Design review of the part built by this model. Coordinates are the model's own, in mm. A direction names the side the tool comes from. Give positions to 0.01 mm unless a question says otherwise; leave off trailing zeros. Loops run counter-clockwise (first coordinate to the right, second up) from the corner with the lowest first, then second, coordinate; pieces in that order, holes last. Notation, with made-up numbers: (35, -3.75) - (84, -3.75) arc R21 cw to (84, 0.25) - close; hole circle Ø2 at (30.5, 66). An arc over 180 degrees is marked (long way). Write each question's results on one line, items separated by ' | '.
from build123d import *

# Parameters (mm, degrees)
CROQUIS1_R                   = 15
SALIENTE_EXTRUIR1_DEPTH      = 3
CROQUIS2_R                   = 8.5
SALIENTE_EXTRUIR2_DEPTH      = 65
CORTAR_EXTRUIR1_DEPTH        = 4
CORTAR_EXTRUIR1_DEPTH_BACK   = 4
CROQUIS3_W                   = 17
CROQUIS3_H                   = 53
CORTAR_EXTRUIR2_DEPTH        = 8
CORTAR_EXTRUIR2_DEPTH_BACK   = 8
CROQUIS4_R                   = 1
CUT_EXTRUDE9_DEPTH           = 2.5
CROQUIS5_W                   = 2
CROQUIS5_H                   = 15
SALIENTE_EXTRUIR3_DEPTH      = 15
CROQUIS6_R                   = 1.5
SALIENTE_EXTRUIR4_DEPTH      = 3
SALIENTE_EXTRUIR5_DEPTH      = 1.5
SALIENTE_EXTRUIR5_DEPTH_BACK = 1.5
REDONDEO2_R                  = 6
CROQUIS8_R                   = 3
CORTAR_EXTRUIR3_DEPTH        = 10
SKETCH1_W                    = 5
SKETCH1_H                    = 5
CUT_EXTRUDE1_DEPTH           = 1
SKETCH2_R                    = 1.25
CUT_EXTRUDE2_DEPTH           = 3
CUT_EXTRUDE10_START          = -1.2
CUT_EXTRUDE10_DEPTH          = 1.2
M3_CLEARANCE_HOLE1_D         = 3.4
M3_CLEARANCE_HOLE1_DEPTH     = 3.978536948
M3_CLEARANCE_HOLE1_TIP       = 1.021463052


with BuildPart() as part:
    # Croquis1 → Saliente-Extruir1 (new body)
    with BuildSketch(Plane(origin=(0, 0, 0), x_dir=(1, 0, 0), z_dir=(0, 1, 0))):
        with Locations(Location((0, 0, 0), (0, 0, 270))):
            Circle(CROQUIS1_R)
    extrude(amount=SALIENTE_EXTRUIR1_DEPTH)

    # Croquis2 → Saliente-Extruir2 (add)
    with BuildSketch(Plane(origin=(0, 3, 0), x_dir=(1, 0, 0), z_dir=(0, 1, 0))):
        with Locations(Location((0, 0, 0), (0, 0, 270))):
            Circle(CROQUIS2_R)
    extrude(amount=SALIENTE_EXTRUIR2_DEPTH)

    # Croquis3 → Cortar-Extruir1 (cut, two sides: drawn at the far end of the back side and taken through both)
    with BuildSketch(Plane.XY.offset(-CORTAR_EXTRUIR1_DEPTH_BACK)):
        with Locations((0, 35.5)):
            Rectangle(CROQUIS3_W, CROQUIS3_H)
    extrude(amount=CORTAR_EXTRUIR1_DEPTH + CORTAR_EXTRUIR1_DEPTH_BACK, mode=Mode.SUBTRACT)

    # Croquis4 → Cortar-Extruir2 (cut, two sides: drawn at the far end of the back side and taken through both)
    with BuildSketch(Plane.XY.offset(-CORTAR_EXTRUIR2_DEPTH_BACK)):
        with Locations(Location((-4, 58.75, 0), (0, 0, 180))):
            Circle(CROQUIS4_R)
        with Locations(Location((4, 58.75, 0), (0, 0, 180))):
            Circle(CROQUIS4_R)
    extrude(amount=CORTAR_EXTRUIR2_DEPTH + CORTAR_EXTRUIR2_DEPTH_BACK, mode=Mode.SUBTRACT)

    # Sketch11 → Cut-Extrude9 (cut)
    with BuildSketch(Plane(origin=(0, 0, 4), x_dir=(-1, 0, 0), z_dir=(0, 0, -1))):
        with BuildLine():
            Line((5.6, 51.5), (5.6, 45))
            Line((5.6, 45), (-5.6, 45))
            Line((-5.6, 45), (-5.6, 51.5))
            ThreePointArc((-5.6, 51.5), (0, 57.1), (5.6, 51.5))
        make_face()
    extrude(amount=-CUT_EXTRUDE9_DEPTH, mode=Mode.SUBTRACT)

    # Croquis5 → Saliente-Extruir3 (add)
    with BuildSketch(Plane.XY):
        with Locations((0, 10.5)):
            Rectangle(CROQUIS5_W, CROQUIS5_H)
    extrude(amount=-SALIENTE_EXTRUIR3_DEPTH)

    # Croquis6 → Saliente-Extruir4 (add)
    with BuildSketch(Plane(origin=(0, 0, -15), x_dir=(-1, 0, 0), z_dir=(0, 0, -1))):
        with BuildLine():
            Line((-10, 0), (10, 0))
            ThreePointArc((10, 0), (12.121320344, 0.878679656), (13, 3))
            Line((13, 3), (13, 15))
            ThreePointArc((13, 15), (12.121320344, 17.121320344), (10, 18))
            Line((10, 18), (-10, 18))
            ThreePointArc((-10, 18), (-12.121320344, 17.121320344), (-13, 15))
            Line((-13, 15), (-13, 3))
            ThreePointArc((-13, 3), (-12.121320344, 0.878679656), (-10, 0))
        make_face()
        with Locations((-10, 7)):
            Circle(CROQUIS6_R, mode=Mode.SUBTRACT)
        with Locations((10, 7)):
            Circle(CROQUIS6_R, mode=Mode.SUBTRACT)
    extrude(amount=-SALIENTE_EXTRUIR4_DEPTH)

    # Croquis7 → Saliente-Extruir5 (add, two sides: drawn at the far end of the back side and taken through both)
    with BuildSketch(Plane(origin=(0, 0, 0), x_dir=(0, 0, -1), z_dir=(1, 0, 0)).offset(-SALIENTE_EXTRUIR5_DEPTH_BACK)):
        Polygon((0, 9), (4, 9), (4, 33), (-4, 33), (-4, 9), align=None)
    extrude(amount=SALIENTE_EXTRUIR5_DEPTH + SALIENTE_EXTRUIR5_DEPTH_BACK)

    # Redondeo2
    redondeo2_edges = [part.edges().sort_by_distance(p)[0] for p in [
        (-1.5, 9, 0),
        (1.5, 9, 0),
    ]]
    fillet(redondeo2_edges, radius=REDONDEO2_R)

    # Croquis8 → Cortar-Extruir3 (cut)
    with BuildSketch(Plane.XZ):
        with Locations(Location((0, 0, 0), (0, 0, 270))):
            Circle(CROQUIS8_R)
    extrude(amount=-CORTAR_EXTRUIR3_DEPTH, mode=Mode.SUBTRACT)

    # Sketch1 → Cut-Extrude1 (cut)
    with BuildSketch(Plane.ZY.offset(1.5)):
        with Locations((0, 20.5)):
            Rectangle(SKETCH1_W, SKETCH1_H)
    extrude(amount=-CUT_EXTRUDE1_DEPTH, mode=Mode.SUBTRACT)

    # Sketch2 → Cut-Extrude2 (cut)
    with BuildSketch(Plane.ZY.offset(0.5)):
        with Locations((0, 20.5)):
            Circle(SKETCH2_R)
    extrude(amount=-CUT_EXTRUDE2_DEPTH, mode=Mode.SUBTRACT)

    # Sketch12 → Cut-Extrude10 (cut)
    with BuildSketch(Plane(origin=(0, 68, 0), x_dir=(1, 0, 0), z_dir=(0, 1, 0)).offset(CUT_EXTRUDE10_START)):
        with BuildLine():
            Line((0, 0.499987676), (-8.4852821, 0.499987676))
            ThreePointArc((-8.4852821, 0.499987676), (-8.499852285, -0.050111177), (-8.478797084, -0.6))
            Line((-8.478797084, -0.6), (0, -0.6))
            Line((0, -0.6), (8.478797084, -0.6))
            ThreePointArc((8.478797084, -0.6), (8.499852285, -0.050111177), (8.4852821, 0.499987676))
            Line((8.4852821, 0.499987676), (0, 0.499987676))
        make_face()
    extrude(amount=CUT_EXTRUDE10_DEPTH, mode=Mode.SUBTRACT)

    # M3 Clearance Hole1
    with Locations(Plane(origin=(0, 68, 0), x_dir=(1, 0, 0), z_dir=(0, 1, 0))):
        with Locations((0, 5), (0, -5)):
            Hole(M3_CLEARANCE_HOLE1_D / 2, depth=M3_CLEARANCE_HOLE1_DEPTH)
            with Locations((0, 0, -(M3_CLEARANCE_HOLE1_DEPTH + M3_CLEARANCE_HOLE1_TIP / 2))):  # 118° drill point
                Cone(0, M3_CLEARANCE_HOLE1_D / 2, M3_CLEARANCE_HOLE1_TIP, mode=Mode.SUBTRACT)


solid = part.part
(1) Insertion check: P1, Ø5, axis at x = 0, z = 0, coming from the -Y side; P2, Ø0.7, axis at y = 48, z = 5, coming from the -X side; P3, Ø2.5, axis at x = -4, y = 58.75, coming from the -Z side. Each pin has a flat end and moves straight along its axis. Give the tip position at first contact, or say it passes through.
Answers below:
P1: y = 10 | P2: x = -7.12 | P3: z = -8.04
(2) Draft analysis for pull direction Y (two halves, no side actions). For faces 5 (the flat face through (13, 9, -14)), 6 (the conical face through (0, 63, -5)), 7 (the cylindrical face through (11.2, 6.1, -13.5)), state which applies: pulls with the +Y half, pulls with the -Y half, needs draft (parallel to the pull), parting line crosses it, or undercut.
Answers below:
face 5: needs draft | face 6: pulls with the +Y half | face 7: undercut
(3) Wall thickness on line 1 along Z through (x, y) = (6.5, 14); line 2 along Z through (x, y) = (0, 65.2); line 3 along Y through (x, z) = (4, -5.5): over which ranges is each line inside the solid? List them lowest first. Write a range as from..to.
Answers below:
line 1: -15..-12, -5.48..-4, 4..5.48 | line 2: -8.5..-6.7, -3.3..3.3, 6.7..8.5 | line 3: 0..57.75, 59.75..68
(4) Take a section at A-A on y = 7. Give the boundary of the cut face in (x, z), plus the area to 3 significant figures.
Answers below:
outline: (-13, -15) - (-11.5, -15) - (-11.5, -12) - (-13, -12) - close; (-8.5, -15) - (8.5, -15) - (8.5, -12) - (1, -12) - (1, -8.44) arc R8.5 ccw (long way) to (-1, -8.44) - (-1, -12) - (-8.5, -12) - close; (11.5, -15) - (13, -15) - (13, -12) - (11.5, -12) - close; hole circle Ø6 at (0, 0) | area: 266 mm2
(5) Take a section at D-D on y = 16. Give the boundary of the cut face in (x, z), plus the area to 3 significant figures.
Answers below:
outline: (-12.83, -15) - (12.83, -15) - (12.83, -12) - (1, -12) - (1, -8.44) arc R8.5 ccw to (7.5, -4) - (1.5, -4) - (1.5, 4) - (7.5, 4) arc R8.5 ccw to (-7.5, 4) - (-1.5, 4) - (-1.5, -4) - (-7.5, -4) arc R8.5 ccw to (-1, -8.44) - (-1, -12) - (-12.83, -12) - close | area: 204 mm2
(6) Take a section at B-B on y = 56. Give the boundary of the cut face in (x, z), plus the area to 3 significant figures.
Answers below:
outline: (-7.5, -4) arc R8.5 ccw to (7.5, -4) - close; (-7.5, 4) - (-3.33, 4) - (-3.33, 6.5) - (3.33, 6.5) - (3.33, 4) - (7.5, 4) arc R8.5 ccw to start | area: 79.5 mm2
(7) Tool access review of faces 1 (the flat face through (0, 36, -4)), 2 (the flat face through (-0.5, 22, -1)), 3 (the flat face through (1.5, 24, 0)), 4 (the flat face through (0, 10, 0)): name each direction out of +Z, -Z, +X, -X, +Y, -Y from which nothing blocks a thin tool from reaching the whole face with its end or side.
Answers below:
face 1: none | face 2: -X | face 3: +X | face 4: -Y
